Input: part model. Units: mm. Frame: model coordinates. Face numbers are marked on the shaded views. A direction names the side the tool comes from. Give positions to 0.01 mm unless a question says otherwise; leave off trailing zeros. Loops run counter-clockwise (first coordinate to the right, second up) from the corner with the lowest first, then second, coordinate; pieces in that order, holes last. Notation, with made-up numbers: M 30,35.5 L 45,35.5 A15 ccw 45,60.5 Z; hole C 11,67.5 d10. An arc over 180 degrees is marked long. One line per item, written item: value. Start each with the question number.
(1) Pin query (flat end, axial travel): P1, Ø1.5, axis at x = -10, y = 16, coming from the +Z side (3 decimals); P2, Ø8.5, axis at x = -5.08, z = 0, coming from the +Y side (3 decimals). Return the tip coordinate at first contact, or that it passes through.
(2) Ray query, line 1 along X through (y, z) = (2.25, 0) (3 decimals); line 2 along Y through (x, z) = (10.16, -10.3) (3 decimals); line 3 along Z through (x, y) = (-10, 23.25) (3 decimals). Return the intervals inside material, ascending. Write a range as from..to.
(3) Pull-direction query (Y, two-part tool) for the marked faces 3, 4 and 5; classes: released by +Y, released by -Y, zero draft, split by the parting line, or undercut.
(4) Section A-A on z = 0. Output: boundary loops of the cut face in (x, y) (3 decimals), plus the area to 3 significant figures.
(5) Section D-D on x = -15. Output: boundary loops of the cut face in (y, z) (3 decimals), plus the area to 3 significant figures.
(6) Section C-C on y = 12.7. Output: boundary loops of the cut face in (x, z) (3 decimals), plus the area to 3 significant figures.
(7) Access query for the marked faces 1 and 2. Directions: +Z, -Z, +X, -X, +Y, -Y. A direction counts if a zero-diameter tool reaches every point of the face in a straight line with its end or side. Return the directions, or none.
(8) Section B-B on x = 10.16. Output: boundary loops of the cut face in (y, z) (3 decimals).
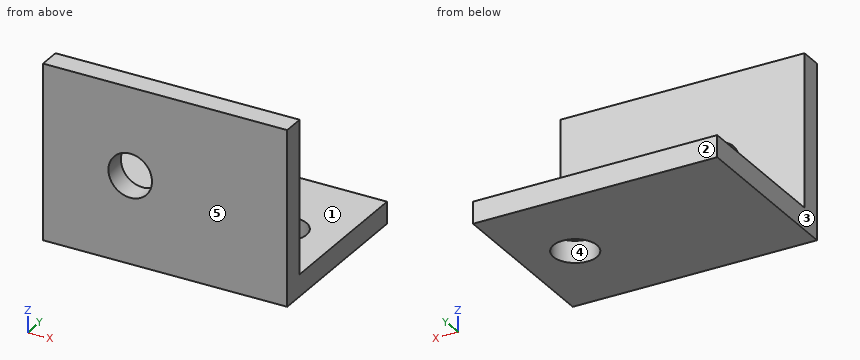
```python
from build123d import *

# Parameters (mm, degrees)
SKETCH1_W           = 35.56
SKETCH1_H           = 25.4
BOSS_EXTRUDE1_DEPTH = 3.175
SKETCH2_W           = 35.56
SKETCH2_H           = 3.175
BOSS_EXTRUDE2_DEPTH = 22.225
SKETCH3_R           = 3.175
CUT_EXTRUDE1_DEPTH  = 3.175
SKETCH4_R           = 3.175
CUT_EXTRUDE2_DEPTH  = 3.175


with BuildPart() as part:
    # Sketch1 → Boss-Extrude1 (new body)
    with BuildSketch(Plane(origin=(0, 0, 0), x_dir=(1, 0, 0), z_dir=(0, 1, 0))):
        Rectangle(SKETCH1_W, SKETCH1_H)
    extrude(amount=BOSS_EXTRUDE1_DEPTH)

    # Sketch2 → Boss-Extrude2 (add)
    with BuildSketch(Plane(origin=(0, 3.175, 0), x_dir=(1, 0, 0), z_dir=(0, 1, 0))):
        with Locations((0, 11.1125)):
            Rectangle(SKETCH2_W, SKETCH2_H)
    extrude(amount=BOSS_EXTRUDE2_DEPTH)

    # Sketch3 → Cut-Extrude1 (cut)
    with BuildSketch(Plane(origin=(0, 3.175, 0), x_dir=(1, 0, 0), z_dir=(0, 1, 0))):
        with Locations(Location((-5.08, 0, 0), (0, 0, 270))):
            Circle(SKETCH3_R)
    extrude(amount=-CUT_EXTRUDE1_DEPTH, mode=Mode.SUBTRACT)

    # Sketch4 → Cut-Extrude2 (cut)
    with BuildSketch(Plane.XY.offset(-9.525)):
        with Locations((10.16, 12.7)):
            Circle(SKETCH4_R)
    extrude(amount=-CUT_EXTRUDE2_DEPTH, mode=Mode.SUBTRACT)


solid = part.part
```
Output values:
1. P1: stops at z = -9.525
1. P2: stops at y = 3.175
2. line 1: x = -17.78..-8.255, -1.905..17.78
2. line 2: y = 0..9.525, 15.875..25.4
2. line 3: z = -12.7..-9.525
3. face 3: zero draft
3. face 4: undercut
3. face 5: released by -Y
4. outline: M -17.78,0 L -8.255,0 L -8.255,3.175 L -17.78,3.175 Z; M -1.905,0 L 17.78,0 L 17.78,3.175 L -1.905,3.175 Z
4. area: 92.7 mm²
5. outline: M 0,-12.7 L 25.4,-12.7 L 25.4,-9.525 L 3.175,-9.525 L 3.175,12.7 L 0,12.7 Z
5. area: 151 mm²
6. outline: M -17.78,-12.7 L 6.985,-12.7 L 6.985,-9.525 L -17.78,-9.525 Z; M 13.335,-12.7 L 17.78,-12.7 L 17.78,-9.525 L 13.335,-9.525 Z
6. area: 92.7 mm²
7. face 1: +Z, +X, -X, +Y
7. face 2: +Z, -Z, +X, -X, +Y
8. outline: M 0,-12.7 L 9.525,-12.7 L 9.525,-9.525 L 3.175,-9.525 L 3.175,12.7 L 0,12.7 Z; M 15.875,-12.7 L 25.4,-12.7 L 25.4,-9.525 L 15.875,-9.525 Z
